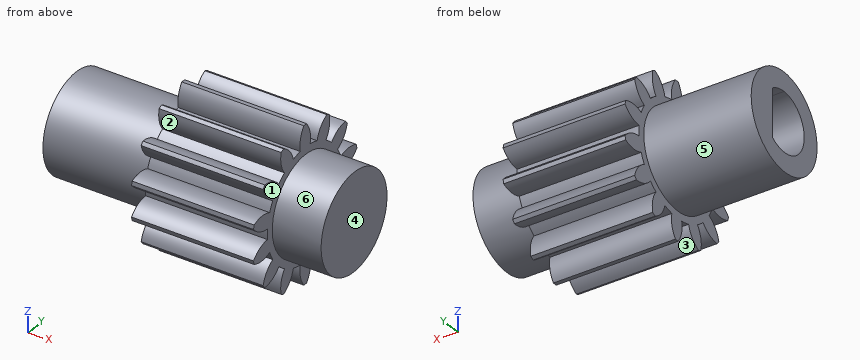
```python
from build123d import *

# Parameters (mm, degrees)
SPUR_START                 = -25.541998066
SPUR_GEAR_AM_OUTLINE_R     = 1.5
SPUR_GEAR_AM_DEPTH         = 14
SPUR_START_2               = -36.542048866
SPUR_GEAR_AM_2_OUTLINE_R   = 5
SPUR_GEAR_AM_2_OUTLINE_R_2 = 1.5
SPUR_GEAR_AM_2_DEPTH       = 11.0000508
SKETCH1_R                  = 10.392655515
CUT_EXTRUDE1_DEPTH         = 1.500223942
SKETCH2_R                  = 5
BOSS_EXTRUDE1_DEPTH        = 5.004484533
SKETCH3_R                  = 1.5
CUT_EXTRUDE2_DEPTH         = 10


# Read off the part's stored shape, not the designer's step: spur gear_am
with BuildPart() as part:
    # spur gear_am outline → spur gear_am (new body)
    with BuildSketch(Plane.YZ.offset(SPUR_START)):
        with BuildLine():
            ThreePointArc((8.934177524, 12.472931761), (8.746459365, 12.38550613), (8.561066896, 12.293251153))
            ThreePointArc((8.561066896, 12.293251153), (8.561742052, 11.085003925), (9.071453323, 9.989533141))
            ThreePointArc((9.071453323, 9.989533141), (8.633086407, 9.672504379), (8.226460402, 9.315673773))
            ThreePointArc((8.226460402, 9.315673773), (7.271876786, 10.0563707), (6.094073075, 10.325889231))
            ThreePointArc((6.094073075, 10.325889231), (5.962877418, 10.165673601), (5.835872509, 10.002115962))
            ThreePointArc((5.835872509, 10.002115962), (6.360719629, 8.913815765), (7.295260575, 8.147986124))
            ThreePointArc((7.295260575, 8.147986124), (7.037859256, 7.672152803), (6.826324883, 7.174231124))
            ThreePointArc((6.826324883, 7.174231124), (5.64489841, 7.427397687), (4.466794227, 7.159195615))
            ThreePointArc((4.466794227, 7.159195615), (4.41810598, 6.957922658), (4.374643512, 6.755456952))
            ThreePointArc((4.374643512, 6.755456952), (5.319710186, 6.002654986), (6.493983512, 5.718148442))
            ThreePointArc((6.493983512, 5.718148442), (6.468529278, 5.177755187), (6.493983512, 4.637361931))
            ThreePointArc((6.493983512, 4.637361931), (5.319710186, 4.352855387), (4.374643512, 3.600053421))
            ThreePointArc((4.374643512, 3.600053421), (4.41810598, 3.397587715), (4.466794227, 3.196314758))
            ThreePointArc((4.466794227, 3.196314758), (5.64489841, 2.928112685), (6.826324883, 3.181279248))
            ThreePointArc((6.826324883, 3.181279248), (7.037859256, 2.68335757), (7.295260575, 2.207524249))
            ThreePointArc((7.295260575, 2.207524249), (6.360719629, 1.441694608), (5.835872509, 0.353394411))
            ThreePointArc((5.835872509, 0.353394411), (5.962877418, 0.189836772), (6.094073075, 0.029621142))
            ThreePointArc((6.094073075, 0.029621142), (7.271876786, 0.299139672), (8.226460402, 1.039836599))
            ThreePointArc((8.226460402, 1.039836599), (8.633086407, 0.683005994), (9.071453323, 0.365977232))
            ThreePointArc((9.071453323, 0.365977232), (8.561742052, -0.729493552), (8.561066896, -1.93774078))
            ThreePointArc((8.561066896, -1.93774078), (8.746459365, -2.029995757), (8.934177524, -2.117421389))
            ThreePointArc((8.934177524, -2.117421389), (9.878402292, -1.363563706), (10.41707606, -0.282040525))
            ThreePointArc((10.41707606, -0.282040525), (10.938256428, -0.427105381), (11.470764997, -0.522538149))
            ThreePointArc((11.470764997, -0.522538149), (11.48683797, -1.730678653), (12.0104685, -2.819564729))
            ThreePointArc((12.0104685, -2.819564729), (12.217529278, -2.822244814), (12.424590055, -2.819564729))
            ThreePointArc((12.424590055, -2.819564729), (12.948220585, -1.730678653), (12.964293559, -0.522538149))
            ThreePointArc((12.964293559, -0.522538149), (13.496802127, -0.427105381), (14.017982495, -0.282040525))
            ThreePointArc((14.017982495, -0.282040525), (14.556656263, -1.363563706), (15.500881031, -2.117421389))
            ThreePointArc((15.500881031, -2.117421389), (15.688599191, -2.029995757), (15.87399166, -1.93774078))
            ThreePointArc((15.87399166, -1.93774078), (15.873316504, -0.729493552), (15.363605233, 0.365977232))
            ThreePointArc((15.363605233, 0.365977232), (15.801972149, 0.683005994), (16.208598153, 1.039836599))
            ThreePointArc((16.208598153, 1.039836599), (17.16318177, 0.299139672), (18.34098548, 0.029621142))
            ThreePointArc((18.34098548, 0.029621142), (18.472181137, 0.189836772), (18.599186046, 0.353394411))
            ThreePointArc((18.599186046, 0.353394411), (18.074338927, 1.441694609), (17.13979798, 2.207524249))
            ThreePointArc((17.13979798, 2.207524249), (17.397199299, 2.68335757), (17.608733673, 3.181279248))
            ThreePointArc((17.608733673, 3.181279248), (18.790160146, 2.928112685), (19.968264329, 3.196314758))
            ThreePointArc((19.968264329, 3.196314758), (20.016952575, 3.397587715), (20.060415044, 3.600053421))
            ThreePointArc((20.060415044, 3.600053421), (19.11534837, 4.352855387), (17.941075043, 4.637361931))
            ThreePointArc((17.941075043, 4.637361931), (17.966529278, 5.177755187), (17.941075043, 5.718148442))
            ThreePointArc((17.941075043, 5.718148442), (19.11534837, 6.002654986), (20.060415044, 6.755456952))
            ThreePointArc((20.060415044, 6.755456952), (20.016952575, 6.957922658), (19.968264329, 7.159195615))
            ThreePointArc((19.968264329, 7.159195615), (18.790160146, 7.427397687), (17.608733673, 7.174231124))
            ThreePointArc((17.608733673, 7.174231124), (17.397199299, 7.672152802), (17.13979798, 8.147986124))
            ThreePointArc((17.13979798, 8.147986124), (18.074338927, 8.913815764), (18.599186046, 10.002115962))
            ThreePointArc((18.599186046, 10.002115962), (18.472181137, 10.165673601), (18.34098548, 10.325889231))
            ThreePointArc((18.34098548, 10.325889231), (17.16318177, 10.0563707), (16.208598153, 9.315673773))
            ThreePointArc((16.208598153, 9.315673773), (15.801972149, 9.672504379), (15.363605233, 9.989533141))
            ThreePointArc((15.363605233, 9.989533141), (15.873316504, 11.085003925), (15.87399166, 12.293251153))
            ThreePointArc((15.87399166, 12.293251153), (15.688599191, 12.38550613), (15.500881031, 12.472931761))
            ThreePointArc((15.500881031, 12.472931761), (14.556656263, 11.719074079), (14.017982495, 10.637550898))
            ThreePointArc((14.017982495, 10.637550898), (13.496802127, 10.782615754), (12.964293559, 10.878048522))
            ThreePointArc((12.964293559, 10.878048522), (12.948220585, 12.086189026), (12.424590055, 13.175075102))
            ThreePointArc((12.424590055, 13.175075102), (12.217529278, 13.177755186), (12.0104685, 13.175075102))
            ThreePointArc((12.0104685, 13.175075102), (11.48683797, 12.086189026), (11.470764997, 10.878048522))
            ThreePointArc((11.470764997, 10.878048522), (10.938256428, 10.782615754), (10.41707606, 10.637550898))
            ThreePointArc((10.41707606, 10.637550898), (9.878402292, 11.719074079), (8.934177524, 12.472931761))
        make_face()
        with Locations((12.217529278, 5.177755186)):
            Circle(SPUR_GEAR_AM_OUTLINE_R, mode=Mode.SUBTRACT)
    extrude(amount=SPUR_GEAR_AM_DEPTH)

    # spur gear_am 2 outline → spur gear_am 2 (add)
    with BuildSketch(Plane.YZ.offset(SPUR_START_2)):
        with Locations((12.217529278, 5.177755186)):
            Circle(SPUR_GEAR_AM_2_OUTLINE_R)
        with Locations((12.217529278, 5.177755186)):
            Circle(SPUR_GEAR_AM_2_OUTLINE_R_2, mode=Mode.SUBTRACT)
    extrude(amount=SPUR_GEAR_AM_2_DEPTH)

    # Sketch1 → Cut-Extrude1 (cut)
    with BuildSketch(Plane(origin=(-11.541998066, 0, 0), x_dir=(0, 0, -1), z_dir=(1, 0, 0))):
        with Locations((-5.177755186, 12.217529278)):
            Circle(SKETCH1_R)
    extrude(amount=-CUT_EXTRUDE1_DEPTH, mode=Mode.SUBTRACT)

    # Sketch2 → Boss-Extrude1 (add)
    with BuildSketch(Plane(origin=(-13.042222007, 0, 0), x_dir=(0, 0, -1), z_dir=(1, 0, 0))):
        with Locations((-5.177755186, 12.217529278)):
            Circle(SKETCH2_R)
    extrude(amount=BOSS_EXTRUDE1_DEPTH)

    # Sketch3 → Cut-Extrude2 (cut)
    with BuildSketch(Plane.ZY.offset(36.542048866)):
        with BuildLine():
            Line((7.682755186, 13.957493358), (2.672755186, 13.957493358))
            ThreePointArc((2.672755186, 13.957493358), (4.266094614, 9.306966617), (8.227755186, 12.217529278))
            ThreePointArc((8.227755186, 12.217529278), (8.088317847, 13.12918985), (7.682755186, 13.957493358))
        make_face()
        with Locations((5.177755186, 12.217529278)):
            Circle(SKETCH3_R, mode=Mode.SUBTRACT)
    extrude(amount=-CUT_EXTRUDE2_DEPTH, mode=Mode.SUBTRACT)


solid = part.part
```
The listing builds one solid part. Answer for the finished solid, in the listing's coordinates (mm). Face numbers are marked on the shaded views. A direction names the side the tool comes from. Give positions to 0.01 mm unless a question says otherwise; leave off trailing zeros. Loops run counter-clockwise (first coordinate to the right, second up) from the corner with the lowest first, then second, coordinate; pieces in that order, holes last. Notation, with made-up numbers: (88, -14.5) - (137, -14.5) arc R30 ccw to (137, 14.5) - close; hole circle Ø2 at (4.25, -3.5). An arc over 180 degrees is marked (long way). Return JSON: item names as keys, results as strings. Group by question number.
1. Given pin 1 Ø5.5 at (x, z) = (-31.5, 6) entering from -Y; pin 2 Ø6 at (x, y) = (-33, 11) entering from -Z; pin 3 Ø1 at (x, y) = (-33.5, 8) entering from -Z, each flat-ended and moving along its own axis, determine where each tip first touches the part or whether it passes through.
2. Find section A-A (z = 4). Write down the section's boundary in (x, y).
3. Determine the mould class of the marked faces 1, 2 and 3 for opening direction Z: pulls with the +Z half, pulls with the -Z half, needs draft (parallel to the pull), parting line crosses it, or undercut.
4. Straight lines are drawn through the part: line 1 (Y direction, x = -19, z = 12); line 2 (Y direction, x = -17, z = -1); line 3 (X direction, y = 6.75, z = 9.75). For each, find the intervals that lie inside material, in ascending order. Write a range as [from, to].
5. Which of the six approach directions +Z, -Z, +X, -X, +Y, -Y give full straight-line access (tool end or side, diameter ignored) to the marked faces 4, 5 and 6?
6. Find section C-C (x = -11.25). Write down the section's boundary in (y, z), then the cut area to 3 significant figures.
7. Find section D-D (x = -31.25). Write down the section's boundary in (y, z), then the cut area to 3 significant figures.
8. Find section B-B (y = 9.5). Write down the section's boundary in (x, z).
Verdict:
{
 "1": {"pin 1": "stops at y = 7.22", "pin 2": "stops at z = 0.18", "pin 3": "stops at z = 1.83"},
 "2": {"outline": "(-36.54, 7.36) - (-25.54, 7.36) - (-25.54, 4.77) - (-13.04, 4.77) - (-13.04, 7.36) - (-8.04, 7.36) - (-8.04, 17.08) - (-13.04, 17.08) - (-13.04, 19.66) - (-25.54, 19.66) - (-25.54, 17.08) - (-36.54, 17.08) - (-36.54, 13.96) - (-26.54, 13.96) - (-26.54, 13.15) - (-13.04, 13.15) - (-13.04, 11.29) - (-26.54, 11.29) - (-26.54, 9.4) - (-36.54, 9.4) - close"},
 "3": {"face 1": "needs draft", "face 2": "undercut", "face 3": "pulls with the -Z half"},
 "4": {"line 1": "y = [8.51, 9.62], [11.47, 12.97], [14.82, 15.92]", "line 2": "y = [8.52, 10.13], [11.41, 13.02], [14.31, 15.92]", "line 3": "x = [-25.54, -13.04]"},
 "5": {"face 4": "+Z, -Z, +X, +Y, -Y", "face 5": "-X", "face 6": "+X"},
 "6": {"outline": "circle Ø10 at (12.22, 5.18)", "area": "78.5 mm^2"},
 "7": {"outline": "circle Ø10 at (12.22, 5.18); hole (13.96, 2.67) - (13.96, 7.68) arc R3.05 ccw (long way) to start", "area": "53.9 mm^2"},
 "8": {"outline": "(-36.54, 0.98) - (-25.54, 0.98) - (-25.54, -1.75) - (-13.04, -1.75) - (-13.04, 0.98) - (-8.04, 0.98) - (-8.04, 9.37) - (-13.04, 9.37) - (-13.04, 12.1) - (-25.54, 12.1) - (-25.54, 9.37) - (-36.54, 9.37) - (-36.54, 6.56) - (-26.54, 6.56) - (-26.54, 3.79) - (-36.54, 3.79) - close"}
}
